```python
from build123d import *

# Parameters (mm, degrees)
BOSS_EXTRUDE1_DEPTH = 1.25
FILLET1_R           = 1


with BuildPart() as part:
    # Sketch1 → Boss-Extrude1 (new, symmetric)
    with BuildSketch(Plane(origin=(0, 0, 0), x_dir=(0, 0, -1), z_dir=(1, 0, 0))):
        with BuildLine():
            Line((7.5, -5), (11.456439237, -5))
            ThreePointArc((11.456439237, -5), (12.5, 0), (11.456439237, 5))
            Line((11.456439237, 5), (-11.456439237, 5))
            ThreePointArc((-11.456439237, 5), (-12.5, 0), (-11.456439237, -5))
            Line((-11.456439237, -5), (-7.5, -5))
            Line((-7.5, -5), (-7.5, 0))
            Line((-7.5, 0), (-6, 0))
            ThreePointArc((-6, 0), (-5.286764074, -2.837274331), (-3.31662479, -5))
            Line((-3.31662479, -5), (-4.153311931, -5))
            Line((-4.153311931, -5), (3.31662479, -5))
            ThreePointArc((3.31662479, -5), (5.286764074, -2.837274331), (6, 0))
            Line((6, 0), (7.5, 0))
            Line((7.5, 0), (7.5, -5))
        make_face()
        with BuildLine():
            ThreePointArc((11.456439237, 5), (0, 12.5), (-11.456439237, 5))
            Line((-11.456439237, 5), (11.456439237, 5))
        make_face()
    extrude(amount=BOSS_EXTRUDE1_DEPTH, both=True)

    # Fillet1
    fillet1_edges = [part.edges().sort_by_distance(p)[0] for p in [
        (0, -5, -3.31662479),
        (0, -5, 3.31662479),
        (0, -5, 7.5),
        (0, -5, 11.456439237),
        (0, -5, -11.456439237),
        (0, -5, -7.5),
    ]]
    fillet(fillet1_edges, radius=FILLET1_R)


solid = part.part
```
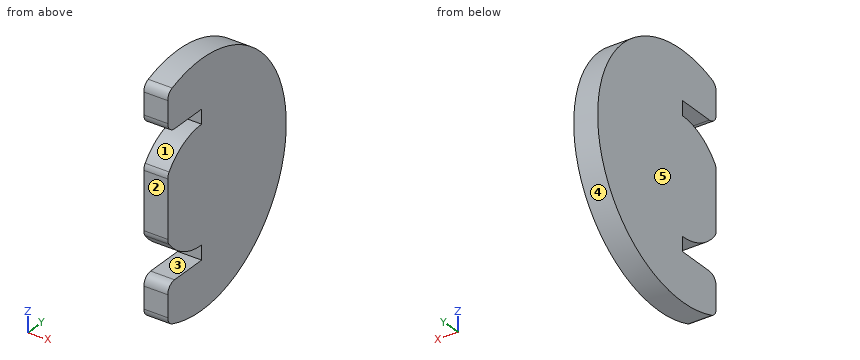
Check sheet for the modelled part. Datum: model origin and axes. Units: mm. Face numbers are marked on the shaded views. A direction names the side the tool comes from. Coordinates: 2 decimals unless noted, no trailing zeros. Order: outer loops, then holes, each group sorted by start corner. A loop starts at its lowest first (then second) coordinate and runs counter-clockwise, first axis right, second up. Notation, with made-up numbers: M 7,50.25 L 26,50.25 A20 cw 26,55.25 Z; hole C 56.25,32 d10. An arc over 180 degrees is marked long. Write each question's results on one line, items separated by ' | '. Start each with the question number.
1. Go/stop test with flat-tipped pins: P1, Ø0.8, axis at x = -0.5, y = -3, coming from the -Z side; P2, Ø0.8, axis at x = -0.5, y = -1, coming from the +Z side. Record where each tip stops, or that it passes through.
2. Material ranges on probe 1 along Z at (x, y) = (0.15, -0.25); probe 2 along Z at (x, y) = (0.8, -1.75); probe 3 along Z at (x, y) = (0.05, 10), recorded low to high.
3. Access from +Z, -Z, +X, -X, +Y, -Y to the whole of each face (thin tool, end or side, straight path). Record for the marked faces 1 and 2.
4. Cross-section at B-B on x = -0.85. Record the cut outline in (y, z), and give its area (3 significant figures).
5. Cross-section at D-D on y = 11.25. Record the cut outline in (x, z), and give its area (3 significant figures).
6. Cross-section at C-C on z = -5.75. Record the cut outline in (x, y), and give its area (3 significant figures).
7. Cross-section at A-A on y = -3.25. Record the cut outline in (x, z).
8. Mould release check, pull along Z, two halves, no side actions. Record for the marked faces 3, 4 and 5: +Z half, -Z half, draft (parallel to the pull), parting line (faces both ways), or undercut.
Checks:
1) P1: stops at z = -12.23 | P2: stops at z = 12.49
2) probe 1: z = -12.5 to -7.5, -5.99 to 5.99, 7.5 to 12.5 | probe 2: z = -12.38 to -7.5, -5.74 to 5.74, 7.5 to 12.38 | probe 3: z = -7.5 to 7.5
3) face 1: +X, -X, -Y | face 2: +Z, -Z, +X, -X, -Y
4) outline: M -5,-10.78 A1 ccw -4.35,-11.72 A12.5 ccw long -4.35,11.72 A1 ccw -5,10.78 L -5,8.5 A1 ccw -4,7.5 L 0,7.5 L 0,6 A6 ccw -4.8,3.6 A1 ccw -5,3 L -5,-3 A1 ccw -4.8,-3.6 A6 ccw 0,-6 L 0,-7.5 L -4,-7.5 A1 ccw -5,-8.5 Z | area: 343 mm²
5) outline: M -1.25,-5.45 L 1.25,-5.45 L 1.25,5.45 L -1.25,5.45 Z | area: 27.2 mm²
6) outline: M -1.25,-1.71 L 1.25,-1.71 L 1.25,11.1 L -1.25,11.1 Z | area: 32.0 mm²
7) outline: M -1.25,-12.07 L 1.25,-12.07 L 1.25,-7.5 L -1.25,-7.5 Z; M -1.25,-5.04 L 1.25,-5.04 L 1.25,5.04 L -1.25,5.04 Z; M -1.25,7.5 L 1.25,7.5 L 1.25,12.07 L -1.25,12.07 Z
8) face 3: undercut | face 4: parting line | face 5: draft
